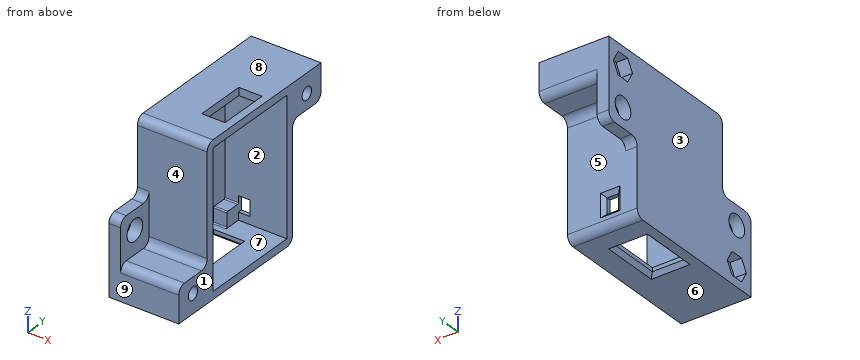
Autodesk Inventor part; units mm, degrees
ref_plane "YZ Plane" through (0, 0, 0) normal (1, 0, 0) x (0, 1, 0)
ref_plane "XZ Plane" through (0, 0, 0) normal (0, 1, 0) x (-1, 0, 0)
ref_plane "XY Plane" through (0, 0, 0) normal (0, 0, 1) x (1, 0, 0)
sketch "Skizze1" plane through (0, 0, 0) normal (1, 0, 0) x (0, 1, 0)
  line L0 (0, 0) -> (30, 0)
  line L1 (30, 0) -> (30, -39)
  line L2 (30, -39) -> (0, -39)
  line L3 (0, -39) -> (0, 0)
  dimension "d0" = 39
  dimension "d1" = 30
extrude "Extrusion1" add sketch "Skizze1" along normal blind 18
shell "Wandung1" thickness 2 removed faces 1 at (18, 10, -13)
sketch "Skizze2" plane through (2, 2, -37) normal (1, 0, 0) x (0, 0, -1)
  line L0 (-35, 26) -> (-35, 0)
  line L1 (-35, 26) -> (-31, 26)
  line L2 (-31, 26) -> (-31, 22)
  line L3 (-31, 22) -> (-35, 22)
  line L4 (-35, 22) -> (-35, 26)
  line L5 (0, 26) -> (0, 0)
  line L6 (0, 26) -> (-4, 26)
  line L7 (-4, 26) -> (-4, 22)
  line L8 (-4, 22) -> (0, 22)
  line L9 (0, 22) -> (0, 26)
  line L10 (0, 0) -> (-4, 0)
  line L11 (-4, 0) -> (-4, 4)
  line L12 (-4, 4) -> (0, 4)
  line L13 (0, 4) -> (0, 0)
  line L14 (-35, 0) -> (0, 0)
  line L15 (-35, 0) -> (-31, 0)
  line L16 (-31, 0) -> (-31, 4)
  line L17 (-31, 4) -> (-35, 4)
  line L18 (-35, 4) -> (-35, 0)
  point P0 (-37, -2)
  point P1 (-35, 4)
  point P2 (-31, 0)
  point P3 (0, 4)
  point P4 (0, 22)
  dimension "d5" = 4
  dimension "d6" = 4
  dimension "d7" = 4
  dimension "d8" = 4
extrude "Extrusion2" add sketch "Skizze2" along normal blind 3.5
fillet "Rundung1" radius 0.3 12 edges at (3.75, 24, -6) (3.75, 24, -2) (3.75, 28, -6) (3.75, 28, -33) (3.75, 24, -33) (3.75, 24, -37) (3.75, 6, -37) (3.75, 6, -33) (3.75, 2, -33) (3.75, 6, -2) (3.75, 6, -6) (3.75, 2, -6)
sketch "Skizze3" plane through (0, 0, -39) normal (0, 0, -1) x (-1, 0, 0)
  line L0 (-10.5, 20) -> (-6.5, 20)
  line L1 (-6.5, 20) -> (-6.5, 11)
  line L2 (-6.5, 11) -> (-10.5, 11)
  line L3 (-10.5, 11) -> (-10.5, 20)
  line L4 (0, 30) -> (-18, 30)
  line L5 (0, 0) -> (-18, 0)
  line L6 (0, 0) -> (0, 30)
  dimension "d12" = 9
  dimension "d13" = 4
  dimension "d15" = 11
  dimension "d16" = 6.5
extrude "Extrusion3" cut sketch "Skizze3" against normal blind 3.5
sketch "Skizze4" plane through (0, 0, -39) normal (0, 0, -1) x (-1, 0, 0)
  line L0 (-11.5, 9) -> (-3.5, 9)
  line L1 (-3.5, 9) -> (-3.5, 22)
  line L2 (-3.5, 22) -> (-11.5, 22)
  line L3 (-11.5, 22) -> (-11.5, 9)
  line L4 (-10.5, 11) -> (-10.5, 20)
  line L5 (-6.5, 11) -> (-10.5, 11)
  point P0 (0, 0)
  dimension "d19" = 1
  dimension "d20" = 8
  dimension "d21" = 13
  dimension "d22" = 2
extrude "Extrusion4" cut sketch "Skizze4" against normal blind 2
sketch "Skizze5" plane through (0, 0, 0) normal (0, 0, 1) x (1, 0, 0)
  line L0 (16, 22) -> (10, 22)
  line L1 (10, 22) -> (10, 9)
  line L2 (10, 9) -> (16, 9)
  line L3 (16, 9) -> (16, 22)
  line L4 (18, 30) -> (18, 0)
  line L5 (0, 30) -> (18, 30)
  point P0 (0, 0)
  dimension "d25" = 13
  dimension "d26" = 6
  dimension "d27" = 2
  dimension "d28" = 8
extrude "Extrusion5" cut sketch "Skizze5" against normal blind 2
sketch "Skizze6" plane through (0, 30, 0) normal (0, 1, 0) x (1, 0, 0)
  line L0 (8.5, 31) -> (5.5, 31)
  line L1 (5.5, 31) -> (5.5, 35)
  line L2 (5.5, 35) -> (8.5, 35)
  line L3 (8.5, 35) -> (8.5, 31)
  line L4 (0, 39) -> (18, 39)
  line L5 (0, 39) -> (0, 0)
  dimension "d31" = 3
  dimension "d32" = 4
  dimension "d33" = 4
  dimension "d34" = 5.5
extrude "Extrusion6" cut sketch "Skizze6" against normal blind 2
chamfer "Fase1" distance 1 angle 45 4 edges at (5.5, 30, -33) (7, 30, -31) (7, 30, -35) (8.5, 30, -33)
chamfer "Fase2" distance 1 angle 45 4 edges at (3.5, 15.5, -39) (7.5, 9, -39) (11.5, 15.5, -39) (7.5, 22, -39)
sketch "Skizze7" plane through (0, 0, 0) normal (-1, 0, 0) x (0, 0, 1)
  line L0 (0, 0) -> (-39, 0)
  line L1 (-39, 30) -> (0, 30)
  line L2 (0, 30) -> (-20, 30)
  line L3 (-20, 30) -> (-20, 40)
  line L4 (-20, 40) -> (0, 40)
  line L5 (0, 40) -> (0, 30)
  line L6 (-39, 0) -> (-19, 0)
  line L7 (-19, 0) -> (-19, -10)
  line L8 (-19, -10) -> (-39, -10)
  line L9 (-39, -10) -> (-39, 0)
  dimension "d43" = 10
  dimension "d44" = 20
  dimension "d45" = 20
  dimension "d46" = 10
extrude "Extrusion7" add sketch "Skizze7" against normal blind 3
sketch "Skizze8" plane through (0, 0, 0) normal (-1, 0, 0) x (0, 0, 1)
  line L0 (-2.1, 36.6743) -> (-2.1, 33.3257)
  line L1 (-2.1, 33.3257) -> (-5, 31.6514)
  line L2 (-5, 31.6514) -> (-7.9, 33.3257)
  line L3 (-7.9, 33.3257) -> (-7.9, 36.6743)
  line L4 (-7.9, 36.6743) -> (-5, 38.3486)
  line L5 (-5, 38.3486) -> (-2.1, 36.6743)
  line L6 (-31.1, -6.6743) -> (-34, -8.3486)
  line L7 (-34, -8.3486) -> (-36.9, -6.6743)
  line L8 (-36.9, -6.6743) -> (-36.9, -3.3257)
  line L9 (-36.9, -3.3257) -> (-34, -1.6514)
  line L10 (-34, -1.6514) -> (-31.1, -3.3257)
  line L11 (-31.1, -3.3257) -> (-31.1, -6.6743)
  line L12 (0, 0) -> (0, 40)
  line L13 (0, 40) -> (-20, 40)
  line L14 (-39, -10) -> (-39, 30)
  line L15 (-39, -10) -> (-19, -10)
  circle A0 centre (-24, -5) radius 2.75
  circle A1 centre (-15, 35) radius 2.75
  line L16 (-19, -10) -> (-19, 0)
  line L17 (-20, 40) -> (-20, 30)
  point P0 (-5, 35)
  point P1 (-34, -5)
  dimension "d49" = 5.8
  dimension "d50" = 5
  dimension "d51" = 5
  dimension "d52" = 5
  dimension "d53" = 5.8
  dimension "d54" = 5
  dimension "d57" = 5.5
  dimension "d58" = 5
  dimension "d59" = 5
  dimension "d60" = 5
  dimension "d61" = 5
extrude "Extrusion8" cut sketch "Skizze8" against normal blind 3
sketch "Skizze9" plane through (3, 0, 0) normal (1, 0, 0) x (0, 0, -1)
  line L0 (19, 0) -> (39, 0)
  line L1 (39, -10) -> (30, -10)
  line L2 (30, -10) -> (30, 0)
  line L3 (30, 0) -> (39, 0)
  line L4 (39, 0) -> (39, -10)
  line L5 (19, -10) -> (39, -10)
  line L6 (0, 0) -> (0, 40)
  line L7 (39, 30) -> (0, 30)
  line L8 (0, 40) -> (9, 40)
  line L9 (9, 40) -> (9, 30)
  line L10 (9, 30) -> (0, 30)
  line L11 (0, 30) -> (0, 40)
  line L12 (39, -10) -> (39, 0)
  dimension "d62" = 9
  dimension "d63" = 9
extrude "Extrusion9" add sketch "Skizze9" along normal blind 15
sketch "Skizze10" plane through (18, 0, 0) normal (1, 0, 0) x (0, 0, -1)
  circle A0 centre (34, -5) radius 1.65
  line L0 (39, -10) -> (39, 30)
  line L1 (30, -10) -> (39, -10)
  circle A1 centre (5, 35) radius 1.65
  line L2 (0, 40) -> (0, 0)
  line L3 (9, 40) -> (0, 40)
  dimension "d66" = 5
  dimension "d67" = 3.3
  dimension "d68" = 5
  dimension "d69" = 5
  dimension "d70" = 5
  dimension "d71" = 3.3
extrude "Extrusion10" cut sketch "Skizze10" against normal blind 19
fillet "Rundung2" radius 2 10 edges at (9, 0, 0) (9, 30, -39) (10.5, -10, -30) (1.5, -10, -19) (1.5, 0, -19) (1.5, 30, -20) (1.5, 40, -20) (10.5, 40, -9) (10.5, 0, -30) (10.5, 30, -9)
properties part number "gehaeuse_wemos"
Work out the finished part from the listing and answer in its coordinate system (mm). Face numbers are marked on the shaded views. A direction names the side the tool comes from. Give positions to 0.01 mm unless a question says otherwise; leave off trailing zeros. Loops run counter-clockwise (first coordinate to the right, second up) from the corner with the lowest first, then second, coordinate; pieces in that order, holes last. Notation, with made-up numbers: (-34.5, 20.5) -> (-19.5, 20.5) arc R36 ccw to (-19.5, 58.5) -> close; hole circle Ø4 at (13, -17.5). An arc over 180 degrees is marked (long way). Put each result on its own line as item: value. Start each with the question number.
Item 1: Find the intervals of material crossed by L1, parallel to Y at x = 10.25, z = -5; L2, parallel to X at y = 18.5, z = -1.5; L3, parallel to Y at x = 15.75, z = -27.5, in increasing order. Write a range as [from, to].
Item 2: Which of the six approach directions +Z, -Z, +X, -X, +Y, -Y give full straight-line access (tool end or side, diameter ignored) to the marked faces 1, 2, 3, 4 and 5?
Item 3: The mould has two halves that part along Z. Classify the marked faces 6, 7, 8 and 9: released by +Z, released by -Z, zero draft, split by the parting line, or undercut.
Item 4: The part is cut by section A-A (x = 6.25). State how many separate pieces and enclosed holes the cut face has, then the cut area to 3 significant figures.
Item 5: The part is cut by section B-B (y = -5). Give the vertices of the cut face in (x, z), then the cut area to 3 significant figures.
Item 6: The part is cut by section C-C (z = -24). Give the vertices of the cut face in (x, y), then the cut area to 4 significant figures.
Item 7: The part is cut by section D-D (y = 20). Give the vertices of the cut face in (x, z).
Item 8: Each of these flat-tipped pins is pushed along its axis until it touches: P1, Ø1.5, axis at y = -4.5, z = -16.5, coming from the -X side; P2, Ø0.8, axis at x = 8, z = -37.5, coming from the +Y side; P3, Ø5, axis at x = 13, z = -5, coming from the -Y side; P4, Ø3.5, axis at x = 2, y = -6, coming from the +Z side. Where does it stop, or does it pass through?
Answers below:
1. L1: [0, 2], [28, 33.35], [36.65, 40]
1. L2: [0, 10], [16, 18]
1. L3: [0, 2], [28, 30]
2. face 1: +Z, -Z, +X, +Y, -Y
2. face 2: +X
2. face 3: +Z, -Z, -X, +Y, -Y
2. face 4: +Z, +X, -Y
2. face 5: -Z, +X, +Y
3. face 6: released by -Z
3. face 7: undercut
3. face 8: released by +Z
3. face 9: zero draft
4. separate pieces: 2
4. enclosed holes: 2
4. area: 385 mm2
5. outline: (0, -39) -> (18, -39) -> (18, -35.65) -> (3, -35.65) -> (3, -36.9) -> (0, -36.9) -> close; (0, -31.1) -> (3, -31.1) -> (3, -32.35) -> (18, -32.35) -> (18, -30) -> (3, -30) -> (3, -26.75) -> (0, -26.75) -> close; (0, -21.25) -> (3, -21.25) -> (3, -19) -> (0, -19) -> close
5. area: 112 mm2
6. outline: (0, -10) -> (3, -10) -> (3, -7.75) -> (0, -7.75) -> close; (0, -2.25) -> (3, -2.25) -> (3, 0) -> (18, 0) -> (18, 2) -> (2, 2) -> (2, 28) -> (18, 28) -> (18, 30) -> (0, 30) -> close
6. area: 137.5 mm2
7. outline: (0, -39) -> (2.5, -39) -> (3.5, -38) -> (3.5, -37) -> (2, -37) -> (2, -2) -> (10, -2) -> (10, 0) -> (0, 0) -> close; (11.5, -38) -> (12.5, -39) -> (18, -39) -> (18, -37) -> (11.5, -37) -> close; (16, -2) -> (18, -2) -> (18, 0) -> (16, 0) -> close
8. P1: through
8. P2: y = 30
8. P3: y = 0
8. P4: z = -19
